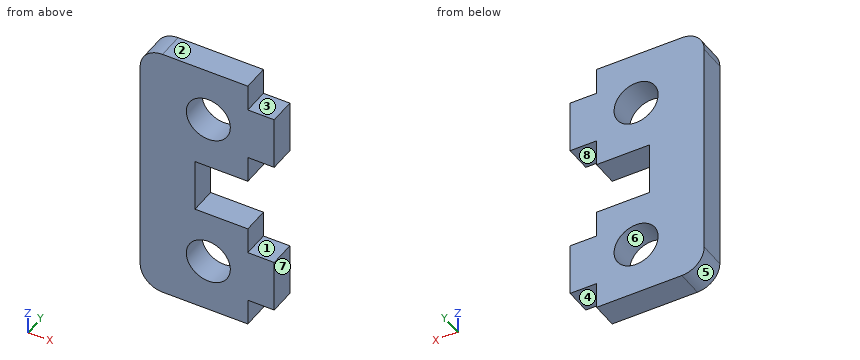
```python
from build123d import *

# Parameters (mm, degrees)
SKETCH1_R           = 5
BOSS_EXTRUDE1_DEPTH = 6


with BuildPart() as part:
    # Sketch1 → Boss-Extrude1 (new body)
    with BuildSketch(Plane(origin=(0, 0, 0), x_dir=(1, 0, 0), z_dir=(0, 1, 0))):
        with BuildLine():
            Line((-21.126722314, 18.92), (-21.126722314, -30.92))
            ThreePointArc((-21.126722314, -30.92), (-19.638824763, -34.512102448), (-16.046722314, -36))
            Line((-16.046722314, -36), (3.332223015, -36))
            Line((3.332223015, -36), (3.332223015, -30))
            Line((3.332223015, -30), (9.332223015, -30))
            Line((9.332223015, -30), (9.332223015, -18))
            Line((9.332223015, -18), (3.332223015, -18))
            Line((3.332223015, -18), (3.332223015, -12))
            Line((3.332223015, -12), (-8.667776985, -12))
            Line((-8.667776985, -12), (-8.667776985, 0))
            Line((-8.667776985, 0), (3.332223015, 0))
            Line((3.332223015, 0), (3.332223015, 6))
            Line((3.332223015, 6), (9.332223015, 6))
            Line((9.332223015, 6), (9.332223015, 18))
            Line((9.332223015, 18), (3.332223015, 18))
            Line((3.332223015, 18), (3.332223015, 24))
            Line((3.332223015, 24), (-16.046722314, 24))
            ThreePointArc((-16.046722314, 24), (-19.638824763, 22.512102448), (-21.126722314, 18.92))
        make_face()
        with Locations(Location((-5.643722664, 11.877299035, 0), (0, 0, 270))):
            Circle(SKETCH1_R, mode=Mode.SUBTRACT)
        with Locations(Location((-5.643722664, -23.877299035, 0), (0, 0, 270))):
            Circle(SKETCH1_R, mode=Mode.SUBTRACT)
    extrude(amount=BOSS_EXTRUDE1_DEPTH)


solid = part.part
```
Geometry check sheet. Reference: the model listing, model coordinates, mm. Face numbers are marked on the shaded views. A direction names the side the tool comes from. Coordinates: 2 decimals unless noted, no trailing zeros. Write each loop counter-clockwise with the first axis right and the second up, starting at its lowest first coordinate (ties: lowest second). Pieces come first, ordered by that corner, then holes. Notation, with made-up numbers: (-28.5, 54) -> (10.5, 54) arc R12 cw to (10.5, 66) -> close; hole circle Ø3 at (-3.75, -4). An arc over 180 degrees is marked (long way). Use CSV: the item, a comma, the result in double quotes. Start each with the question number.
Item 1: Mould release check, pull along Z, two halves, no side actions. Record for the marked faces 5, 6, 7 and 8: released by +Z, released by -Z, zero draft, split by the parting line, or undercut.
Item 2: Cross-section at A-A, the plane x = 4.5. Record the cut outline in (y, z).
Item 3: Thickness scan on line 1 (Z direction, x = 8.5, y = 3.35); line 2 (Z direction, x = -6, y = 0.95); line 3 (Z direction, x = -9, y = 0.75). Record the ranges inside material, lowest first.
Item 4: Cross-section at B-B, the plane z = 26. Record the cut outline in (x, y).
Item 5: Depth check by flat-ended pin: pin 1 Ø1.8 at (y, z) = (3, 8) entering from +X; pin 2 Ø3 at (x, y) = (5.5, 1.5) entering from +Z; pin 3 Ø3 at (y, z) = (3, 13.5) entering from +X; pin 4 Ø3 at (x, z) = (-2, -3) entering from -Y. Enter the tip coordinate at first touch or a pass-through.
Item 6: Cross-section at C-C, the plane x = -8. Record the cut outline in (y, z).
Item 7: Cross-section at D-D, the plane y = 3.25. Record the cut outline in (x, z).
Item 8: Set-up check for the marked faces 1, 2, 3 and 4: record each of +Z, -Z, +X, -X, +Y, -Y from which the full face is reachable in a straight line by a thin tool's end or side.
Answers:
1,face 5,"released by -Z"
1,face 6,"undercut"
1,face 7,"zero draft"
1,face 8,"undercut"
2,outline,"(0, -18) -> (6, -18) -> (6, -6) -> (0, -6) -> close; (0, 18) -> (6, 18) -> (6, 30) -> (0, 30) -> close"
3,line 1,"-18 to -6, 18 to 30"
3,line 2,"-24 to -16.86, -6.89 to 0, 12 to 18.89, 28.86 to 36"
3,line 3,"-24 to -15.58, -8.17 to 20.17, 27.58 to 36"
4,outline,"(-21.13, 0) -> (-10.17, 0) -> (-10.17, 6) -> (-21.13, 6) -> close; (-1.12, 0) -> (9.33, 0) -> (9.33, 6) -> (-1.12, 6) -> close"
5,pin 1,"x = -8.67"
5,pin 2,"z = 30"
5,pin 3,"x = 3.33"
5,pin 4,"y = 0"
6,outline,"(0, -24) -> (6, -24) -> (6, -16.29) -> (0, -16.29) -> close; (0, -7.47) -> (6, -7.47) -> (6, 0) -> (0, 0) -> close; (0, 12) -> (6, 12) -> (6, 19.47) -> (0, 19.47) -> close; (0, 28.29) -> (6, 28.29) -> (6, 36) -> (0, 36) -> close"
7,outline,"(-21.13, -18.92) arc R5.08 ccw to (-16.05, -24) -> (3.33, -24) -> (3.33, -18) -> (9.33, -18) -> (9.33, -6) -> (3.33, -6) -> (3.33, 0) -> (-8.67, 0) -> (-8.67, 12) -> (3.33, 12) -> (3.33, 18) -> (9.33, 18) -> (9.33, 30) -> (3.33, 30) -> (3.33, 36) -> (-16.05, 36) arc R5.08 ccw to (-21.13, 30.92) -> close; hole circle Ø10 at (-5.64, -11.88); hole circle Ø10 at (-5.64, 23.88)"
8,face 1,"+X, +Y, -Y"
8,face 2,"+Z, +X, -X, +Y, -Y"
8,face 3,"+Z, +X, +Y, -Y"
8,face 4,"-Z, +X, +Y, -Y"
